Read the model definition and answer for the solid it produces. Units are mm, in the model's axes. A direction names the side the tool comes from. Round coordinates to 2 decimals unless told otherwise and drop trailing zeros. Write each loop counter-clockwise with the first axis right and the second up, starting at its lowest first coordinate (ties: lowest second). Pieces come first, ordered by that corner, then holes. Notation, with made-up numbers: (5.25, 7) - (26.25, 7) arc R12 cw to (26.25, 14) - close; hole circle Ø11 at (67.5, 87.25). An arc over 180 degrees is marked (long way). Answer as CSV lines item,"result". Start each with the question number.
1) For a pull along X with two mould halves and no side action, classify faces 6 (the flat face through (42, 52.1, 6)), 7 (the flat face through (66.5, 2, 6)), 8 (the flat face through (23.1, 13, 10)) as +X half, -X half, draft (parallel to the pull), parting line (faces both ways), or undercut.
2) Find section B-B on x = 5. Determine the outline of the cut face in (y, z), then the cut area to 3 significant figures.
3) Consider line 1 along X through (y, z) = (14, 16.25); line 2 along Y through (x, z) = (45, 2.5); line 3 along Y through (x, z) = (25.5, 10). Determine where each line is inside the solid, lowest interval first.
4) Which of the six approach directions +Z, -Z, +X, -X, +Y, -Y give full straight-line access (tool end or side, diameter ignored) to faces 1 (the flat face through (56, 8.9, 10)), 2 (the flat face through (51.2, 13, 10)), 3 (the flat face through (20.7, 13, 10)), 4 (the flat face through (16, 16.9, 10)), 5 (the flat face through (46, 1.2, 6))?
5) Each of these flat-tipped pins is pushed along its axis until it touches: pin 1 (5 mm diameter, centred on x = 29.5, z = 10, fed in from +Y); pin 2 (4 mm diameter, centred on y = 13, z = 10, fed in from -X); pin 3 (2.5 mm diameter, centred on y = 12, z = 6, fed in from +X). Where does it stop, or does it pass through?
6) Find section D-D on x = 47. Determine the outline of the cut face in (y, z).
7) Find section A-A on z = 12.5. Determine the outline of the cut face in (x, y).
8) Find section C-C on z = 7. Determine the outline of the cut face in (x, y), then the cut area to 3 significant figures.
from build123d import *

# Parameters (mm, degrees)
SKETCH1_W           = 68.6
SKETCH1_H           = 53.3
BOSS_EXTRUDE1_DEPTH = 1.6
SKETCH2_W           = 10.1
SKETCH2_H           = 8
SKETCH2_W_2         = 9.9
SKETCH2_W_3         = 9.8
BOSS_EXTRUDE2_DEPTH = 18.1
SKETCH3_W           = 8
SKETCH3_H           = 7.3
BOSS_EXTRUDE3_DEPTH = 11.6
SKETCH4_W           = 49
SKETCH4_H           = 2.6
SKETCH4_W_2         = 39.5
BOSS_EXTRUDE4_DEPTH = 10.1


with BuildPart() as part:
    # Sketch1 → Boss-Extrude1 (new body)
    with BuildSketch(Plane.XY):
        with Locations((34.3, 26.65)):
            Rectangle(SKETCH1_W, SKETCH1_H)
    extrude(amount=BOSS_EXTRUDE1_DEPTH)

    # Sketch2 → Boss-Extrude2 (add)
    with BuildSketch(Plane.XY):
        with Locations((15.65, 12.9)):
            Rectangle(SKETCH2_W, SKETCH2_H)
        with Locations((28.05, 12.9)):
            Rectangle(SKETCH2_W_2, SKETCH2_H)
        with Locations((43.8, 12.9)):
            Rectangle(SKETCH2_W_3, SKETCH2_H)
        with Locations((56.25, 12.9)):
            Rectangle(SKETCH2_W, SKETCH2_H)
    extrude(amount=BOSS_EXTRUDE2_DEPTH)

    # Sketch3 → Boss-Extrude3 (add)
    with BuildSketch(Plane.XY):
        with Locations((4, 19.35)):
            Rectangle(SKETCH3_W, SKETCH3_H)
    extrude(amount=BOSS_EXTRUDE3_DEPTH)

    # Sketch4 → Boss-Extrude4 (add)
    with BuildSketch(Plane.XY):
        with Locations((42, 50.8)):
            Rectangle(SKETCH4_W, SKETCH4_H)
        with Locations((46.75, 2.5)):
            Rectangle(SKETCH4_W_2, SKETCH4_H)
    extrude(amount=BOSS_EXTRUDE4_DEPTH)


solid = part.part
Check values:
1,face 6,"draft"
1,face 7,"+X half"
1,face 8,"undercut"
2,outline,"(0, 0) - (53.3, 0) - (53.3, 1.6) - (23, 1.6) - (23, 11.6) - (15.7, 11.6) - (15.7, 1.6) - (0, 1.6) - close"
2,area,"158 mm^2"
3,line 1,"x = 10.6 to 20.7, 23.1 to 33, 38.9 to 48.7, 51.2 to 61.3"
3,line 2,"y = 1.2 to 3.8, 8.9 to 16.9, 49.5 to 52.1"
3,line 3,"y = 8.9 to 16.9, 49.5 to 52.1"
4,face 1,"+Z, +X, -X"
4,face 2,"+Z"
4,face 3,"+Z, -Y"
4,face 4,"+Z, +X"
4,face 5,"+Z, +X, -X, -Y"
5,pin 1,"stops at y = 52.1"
5,pin 2,"stops at x = 10.6"
5,pin 3,"stops at x = 61.3"
6,outline,"(0, 0) - (53.3, 0) - (53.3, 1.6) - (52.1, 1.6) - (52.1, 10.1) - (49.5, 10.1) - (49.5, 1.6) - (16.9, 1.6) - (16.9, 18.1) - (8.9, 18.1) - (8.9, 1.6) - (3.8, 1.6) - (3.8, 10.1) - (1.2, 10.1) - (1.2, 1.6) - (0, 1.6) - close"
7,outline,"(10.6, 8.9) - (20.7, 8.9) - (20.7, 16.9) - (10.6, 16.9) - close; (23.1, 8.9) - (33, 8.9) - (33, 16.9) - (23.1, 16.9) - close; (38.9, 8.9) - (48.7, 8.9) - (48.7, 16.9) - (38.9, 16.9) - close; (51.2, 8.9) - (61.3, 8.9) - (61.3, 16.9) - (51.2, 16.9) - close"
8,outline,"(0, 15.7) - (8, 15.7) - (8, 23) - (0, 23) - close; (10.6, 8.9) - (20.7, 8.9) - (20.7, 16.9) - (10.6, 16.9) - close; (17.5, 49.5) - (66.5, 49.5) - (66.5, 52.1) - (17.5, 52.1) - close; (23.1, 8.9) - (33, 8.9) - (33, 16.9) - (23.1, 16.9) - close; (27, 1.2) - (66.5, 1.2) - (66.5, 3.8) - (27, 3.8) - close; (38.9, 8.9) - (48.7, 8.9) - (48.7, 16.9) - (38.9, 16.9) - close; (51.2, 8.9) - (61.3, 8.9) - (61.3, 16.9) - (51.2, 16.9) - close"
8,area,"608 mm^2"
